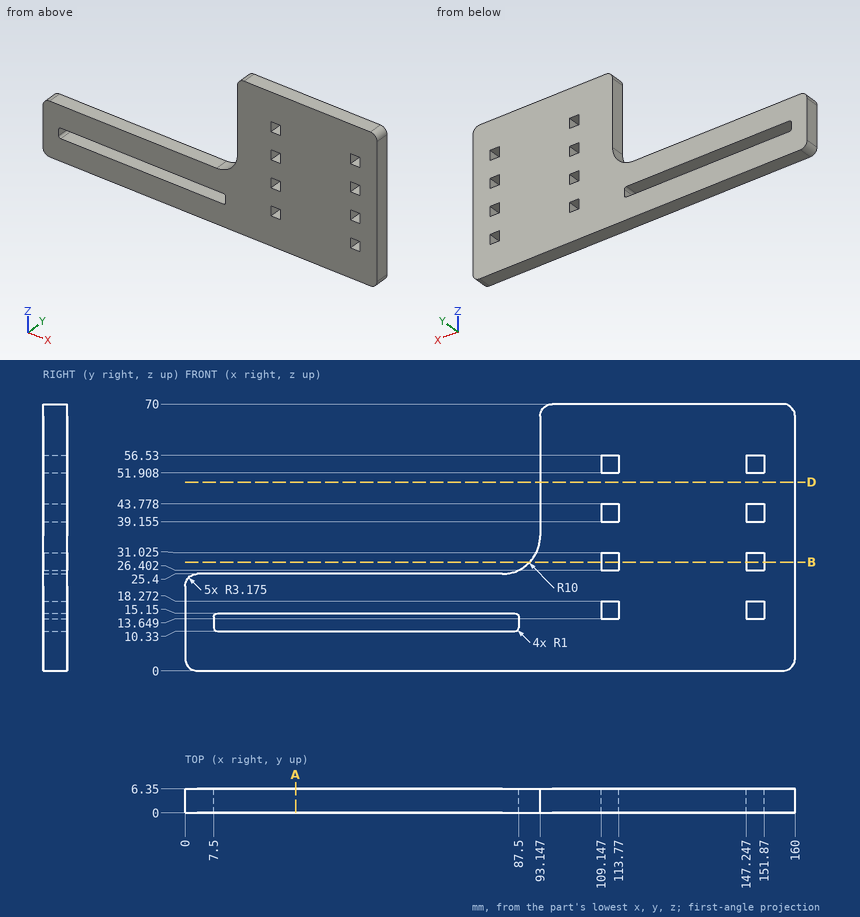
Design review of the part shown in the three views and the two pictorial views. Dimensions are in mm from the part's minimum x, y and z. Give positions to 0.01 mm unless a question says otherwise; leave off trailing zeros. Loops run counter-clockwise (first coordinate to the right, second up) from the corner with the lowest first, then second, coordinate; pieces in that order, holes last. Notation, with made-up numbers: (0, -39) -> (51, -39) arc R27 cw to (51, -6) -> close; hole circle Ø2 at (68, 31.5). An arc over 180 degrees is marked (long way). Answer as a JSON object with one key per item and string values. Group by question number.
Q1. Take a section at D-D (z = 49.5). Write out the cut boundary in (x, y).
Q2. Take a section at A-A (x = 29). Write out the cut boundary in (y, z), plus the area to 3 significant figures.
Q3. Insertion check: pin 1 (3.5 mm diameter, centred on x = 112, y = 2.5, fed in from -Z); pin 2 (1.4 mm diameter, centred on y = 2.5, z = 29, fed in from -X); pin 3 (2.5 mm diameter, centred on y = 2, z = 53.5, fed in from -X). Each pin has a flat end and moves straight along its axis. Give the tip position at first contact, or say it passes through.
Q4. Wall thickness on line 1 along X through (y, z) = (4.5, 14); line 2 along Z through (x, y) = (20.5, 2); line 3 along X through (y, z) = (6, 40): over which ranges is each line inside the solid? List them lowest first.
Q5. Take a section at B-B (z = 28.5). State how many separate pieces and enclosed holes the cut face has, plus the area to 3 significant figures.
Answer below:
{
 "1": {"outline": "(93.15, 0) -> (160, 0) -> (160, 6.35) -> (93.15, 6.35) -> close"},
 "2": {"outline": "(0, 0) -> (6.35, 0) -> (6.35, 10.33) -> (0, 10.33) -> close; (0, 15.15) -> (6.35, 15.15) -> (6.35, 25.4) -> (0, 25.4) -> close", "area": "131 mm2"},
 "3": {"pin 1": "stops at z = 0", "pin 2": "stops at x = 90.19", "pin 3": "stops at x = 93.15"},
 "4": {"line 1": "x = 0 to 7.5, 87.5 to 109.15, 113.77 to 147.25, 151.87 to 160", "line 2": "z = 0 to 10.33, 15.15 to 25.4", "line 3": "x = 93.15 to 109.15, 113.77 to 147.25, 151.87 to 160"},
 "5": {"separate pieces": "3", "enclosed holes": "0", "area": "383 mm2"}
}
